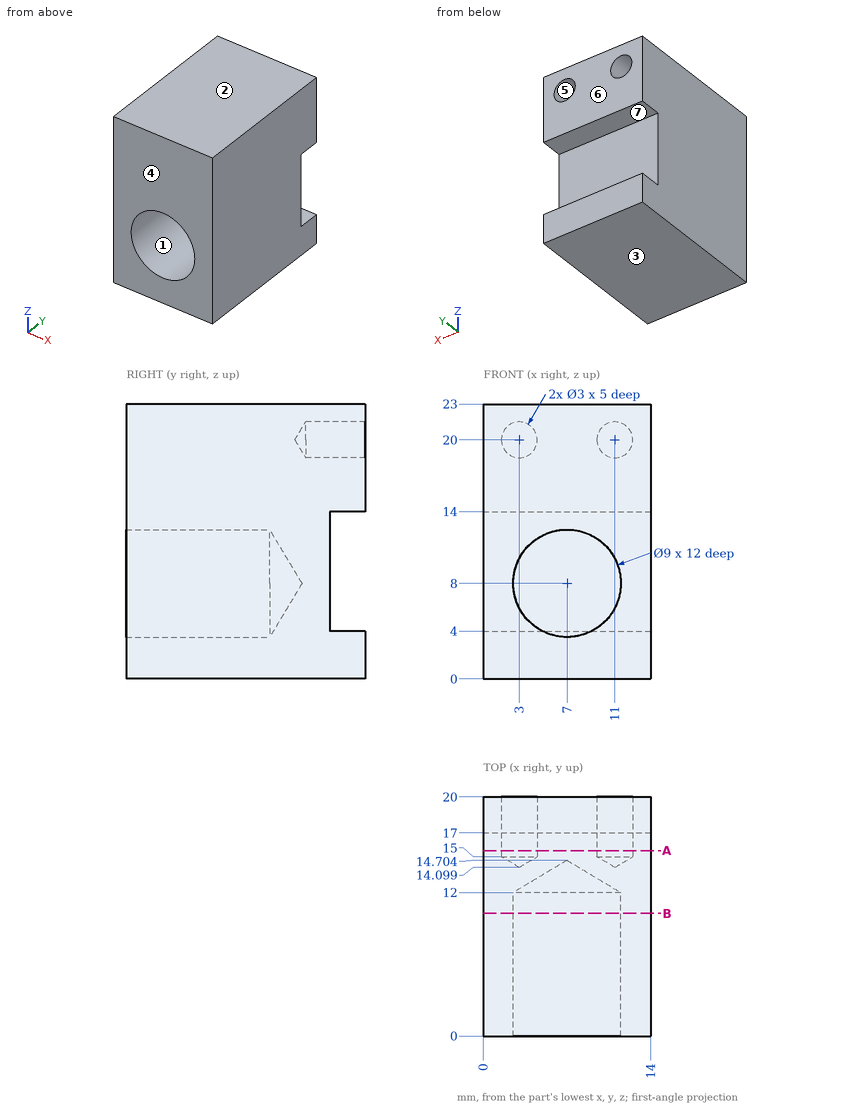
Design review of the part shown in the three views and the two pictorial views. Dimensions are in mm from the part's minimum x, y and z. A direction names the side the tool comes from. Coordinates: 2 decimals unless noted, no trailing zeros. Loops run counter-clockwise (first coordinate to the right, second up) from the corner with the lowest first, then second, coordinate; pieces in that order, holes last.
Q1. Tool access review of the marked faces 5, 6 and 7: name each direction out of +Z, -Z, +X, -X, +Y, -Y from which nothing blocks a thin tool from reaching the whole face with its end or side.
Reported:
face 5: +Y
face 6: +Z, -Z, +X, -X, +Y
face 7: +X, -X, +Y
Q2. We need section A-A on y = 15.5. State the section outline as (x, z) points, and give its area (3 significant figures).
Reported:
outline: (0, 0) - (14, 0) - (14, 23) - (0, 23) - close; hole circle Ø3 at (3, 20); hole circle Ø3 at (11, 20)
area: 308 mm2
Q3. We need section B-B on y = 10.25. State the section outline as (x, z) points.
Reported:
outline: (0, 0) - (14, 0) - (14, 23) - (0, 23) - close; hole circle Ø9 at (7, 8)
Q4. The part is to be moulded in two halves that separate along Z. For the marked faces 1, 2, 3 and 4, say which applies: +Z half, -Z half, draft (parallel to the pull), parting line (faces both ways), or undercut.
Reported:
face 1: undercut
face 2: +Z half
face 3: -Z half
face 4: draft
Q5. To check wall thickness, follow line 1 (X direction, y = 18.05, z = 20); line 2 (Z direction, x = 3, y = 17.55); line 3 (Z direction, x = 7, y = 2). State the ranges of each line that lie inside material, in increasing order.
Reported:
line 1: x = 0 to 1.5, 4.5 to 9.5, 12.5 to 14
line 2: z = 0 to 4, 14 to 18.5, 21.5 to 23
line 3: z = 0 to 3.5, 12.5 to 23
Q6. For pin 1 (5.5 mm diameter, centred on x = 7, z = 8, fed in from -Y); pin 2 (2 mm diameter, centred on x = 4, z = 10, fed in from +Y), all flat-tipped, find the tip position at first contact; note any pin that passes through.
Reported:
pin 1: stops at y = 13.05
pin 2: stops at y = 17
